Part model, mm, in its own coordinate system. Round coordinates to 2 decimals unless told otherwise and drop trailing zeros. Write each loop counter-clockwise with the first axis right and the second up, starting at its lowest first coordinate (ties: lowest second). Pieces come first, ordered by that corner, then holes. Notation, with made-up numbers: M 41.5,30.5 L 47.5,30.5 A25 ccw 47.5,66.5 Z; hole C 83,-2.5 d6. An arc over 180 degrees is marked long. Answer as a JSON object with one key per item and string values. Group by question number.
1. Drop flat-ended pins along their axis: pin 1 (1 mm diameter, centred on y = 14, z = 54, fed in from +X); pin 2 (5 mm diameter, centred on x = -6.5, z = 74.5, fed in from -Y); pin 3 (6 mm diameter, centred on y = 9, z = 157.5, fed in from -X); pin 4 (1.3 mm diameter, centred on x = 70, z = 90, fed in from -Y). Give the stop position or say it passes through.
2. Band-saw the part on C-C, the plane x = 0.5. Write the cut outline in (y, z).
3. Drill centre lines: line 1 (X direction, y = 36, z = 64); line 2 (Y direction, x = 5, z = 82); line 3 (X direction, y = 28.5, z = 148). Where is each one in solid material? Low to high. Write a range as from..to.
4. Band-saw the part on B-B, the plane y = 9. Write the cut outline in (x, z).
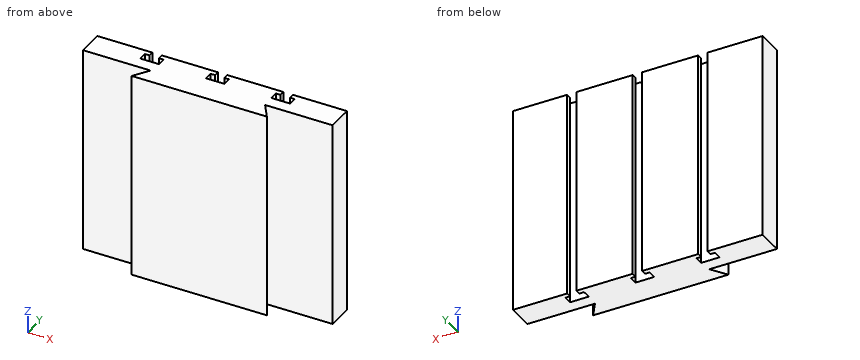
from build123d import *

# Parameters (mm, degrees)
EXTRUDE_1_DEPTH     = 200
CUT_EXTRUDE_1_DEPTH = 201


with BuildPart() as part:
    # Эскиз1 → Бобышка-Вытянуть1 (new body)
    with BuildSketch(Plane.XY):
        Polygon((0, 0), (65, 0), (55, 15), (120, 15), (120, 40), (0, 40), (-120, 40), (-120, 15), (-55, 15), (-65, 0), align=None)
    extrude(amount=EXTRUDE_1_DEPTH)

    # Эскиз2 → Вырез-Вытянуть1 (cut, through all)
    with BuildSketch(Plane.XY.offset(200)):
        Polygon((-8.573821021, 27), (9.426178979, 27), (9.426178979, 35), (4.926178979, 35), (4.926178979, 40), (-4.073821021, 40), (-4.073821021, 35), (-8.573821021, 35), align=None)
        Polygon((54.426178979, 27), (72.426178979, 27), (72.426178979, 35), (67.926178979, 35), (67.926178979, 40), (58.926178979, 40), (58.926178979, 35), (54.426178979, 35), align=None)
        Polygon((-71.573821021, 27), (-53.573821021, 27), (-53.573821021, 35), (-58.073821021, 35), (-58.073821021, 40), (-67.073821021, 40), (-67.073821021, 35), (-71.573821021, 35), align=None)
    extrude(amount=-CUT_EXTRUDE_1_DEPTH, mode=Mode.SUBTRACT)


solid = part.part
Worked answers:
{
 "1": {"pin 1": "stops at x = 56", "pin 2": "stops at y = 0", "pin 3": "stops at x = -61", "pin 4": "stops at y = 15"},
 "2": {"outline": "M 0,0 L 27,0 L 27,200 L 0,200 Z"},
 "3": {"line 1": "x = -120..-67.07, -58.07..-4.07, 4.93..58.93, 67.93..120", "line 2": "y = 0..27, 35..40", "line 3": "x = -120..-71.57, -53.57..-8.57, 9.43..54.43, 72.43..120"},
 "4": {"outline": "M -59,0 L 59,0 L 59,200 L -59,200 Z"}
}
